Verification items for the finished model (mm, model axes). A direction names the side the tool comes from. Round coordinates to 2 decimals unless told otherwise and drop trailing zeros. Write each loop counter-clockwise with the first axis right and the second up, starting at its lowest first coordinate (ties: lowest second). Pieces come first, ordered by that corner, then holes. Notation, with made-up numbers: M 36,60.5 L 85,60.5 A24 ccw 85,81.5 Z; hole C 11.5,-34 d7. An arc over 180 degrees is marked long. One line per item, written item: value. Start each with the question number.
Item 1: Gauge pin test, flat ends, axial feed: pin 1 (4 mm diameter, centred on y = -33.5, z = 19.5, fed in from -X); pin 2 (2 mm diameter, centred on x = -33, z = 20, fed in from +Y); pin 3 (2 mm diameter, centred on y = -28.5, z = 12, fed in from -X); pin 4 (2 mm diameter, centred on y = -20.5, z = 19, fed in from -X). Record the tip position at first contact, or that the pin passes through.
Item 2: Section check A-A, the plane z = 17.25. Record the cut outline in (x, y), then the cut area to 3 significant figures.
Item 3: Tool access check on faces 1 (the face through (-35, -40.5, 18)), 2 (the face through (-36, -51.75, 15)). Record the directions out of +Z, -Z, +X, -X, +Y, -Y that give a thin tool (end or side, any length) a straight path to the whole face; none if there is none.
Item 4: Section check C-C, the plane z = 11.25. Record the cut outline in (x, y).
Item 5: Section check D-D, the plane y = -6.5. Record the cut outline in (x, z).
Item 6: Thickness scan on probe 1 along Y at (x, z) = (-35.75, 19.5); probe 2 along Z at (x, y) = (-36, -10); probe 3 along X at (y, z) = (-44.5, 15). Record the ranges inside material, lowest first. Write a range as from..to.
Item 7: Section check B-B, the plane x = -35.5. Record the cut outline in (y, z).
from build123d import *

# Parameters (mm, degrees)
F0_R     = 6.635
F1_DEPTH = 5.5
F2_R     = 3.9935
F3_DEPTH = 35
F4_R     = 3
F5_DEPTH = 11.25


with BuildPart() as f1:
    # F0 (on Front) → F1 (new body)
    with BuildSketch(Plane.XZ):
        with Locations((-35.828222, 14.797199)):
            Circle(F0_R)
    extrude(amount=F1_DEPTH)

    # F2 (on face) → F3 (join)
    with BuildSketch(Plane.XZ.offset(5.5)):
        with Locations((-35.828222, 14.797199)):
            Circle(F2_R)
    extrude(amount=F3_DEPTH)

    # F4 (on face) → F5 (join)
    with BuildSketch(Plane.XZ.offset(40.5)):
        with Locations((-35.828222, 14.797199)):
            Circle(F4_R)
    extrude(amount=F5_DEPTH)


solid = f1.part
Response values:
1. pin 1: stops at x = -38.77
1. pin 2: stops at y = 0
1. pin 3: stops at x = -39.39
1. pin 4: stops at x = -38.21
2. outline: M -41.99,-5.5 L -38.98,-5.5 L -38.98,-40.5 L -37.56,-40.5 L -37.56,-51.75 L -34.1,-51.75 L -34.1,-40.5 L -32.68,-40.5 L -32.68,-5.5 L -29.66,-5.5 L -29.66,0 L -41.99,0 Z
2. area: 327 mm2
3. face 1: -Y
3. face 2: +Z, -Z, +X, -X, -Y
4. outline: M -41.44,-5.5 L -37.66,-5.5 L -37.66,-40.5 L -33.99,-40.5 L -33.99,-5.5 L -30.22,-5.5 L -30.22,0 L -41.44,0 Z
5. outline: C -35.83,14.8 d7.99
6. probe 1: y = -5.5..0
6. probe 2: z = 10.81..18.79
6. probe 3: x = -38.82..-32.84
7. outline: M -51.75,11.82 L -40.5,11.82 L -40.5,10.82 L -5.5,10.82 L -5.5,8.17 L 0,8.17 L 0,21.42 L -5.5,21.42 L -5.5,18.78 L -40.5,18.78 L -40.5,17.78 L -51.75,17.78 Z
